For this review, take the finished solid that the model builds, in its own axes (mm). A direction names the side the tool comes from. Round coordinates to 2 decimals unless told otherwise and drop trailing zeros. Write each loop counter-clockwise with the first axis right and the second up, starting at its lowest first coordinate (ties: lowest second). Pieces come first, ordered by that corner, then holes. Notation, with made-up numbers: (65, 82.25) - (115, 82.25) arc R29 ccw to (115, 120.25) - close; hole circle Ø4 at (-8.75, 4). An arc over 180 degrees is marked (long way). One line per item, written item: value. Start each with the question number.
Q1. Add section B-B on x = -2.25. Write out the cut boundary in (y, z), and give its area (3 significant figures).
Q2. Tool access review of faces 4 (the face through (0, 0, -30)), 5 (the face through (0, 30, -60)): name each direction out of +Z, -Z, +X, -X, +Y, -Y from which nothing blocks a thin tool from reaching the whole face with its end or side.
Q3. For probe 1 along Y at (x, z) = (2, 0); probe 2 along Z at (x, y) = (-6, 80.5); probe 3 along Z at (x, y) = (-0.5, 57), list the stretches that pass through material, from the lowest coordinate up.
Q4. Mouldability with a two-part tool opening along Y and no side actions: class faces 1 (the face through (-6.35, 35, 28)), 2 (the face through (0.089, 119.985, -1.319)), 3 (the face through (-0.089, 80.275, 22.111)) as +Y half, -Y half, draft (parallel to the pull), parting line (faces both ways), or undercut.
Q5. Add section C-C on z = -10. Write out the cut boundary in (x, y).
Q6. Clearance check with flat-ended pins moving along their axes: pin 1 Ø1 at (x, y) = (-4, 81.5) entering from +Z (3 decimals); pin 2 Ø6.5 at (x, z) = (-0.5, -40) entering from -Y. State where each tip first meets the part, or that it passes through.
Q7. Add section D-D on z = 50. Write out the cut boundary in (x, y), and give its area (3 significant figures).
Q8. Add section A-A on y = 46.5. Write out the cut boundary in (x, z), and give its area (3 significant figures).
```python
from build123d import *

# Parameters (mm, degrees)
SKETCH1_R           = 30
BOSS_EXTRUDE1_DEPTH = 6.35


with BuildPart() as part:
    # Sketch1 → Boss-Extrude1 (new body, symmetric)
    with BuildSketch(Plane(origin=(0, 0, 0), x_dir=(0, 0, -1), z_dir=(1, 0, 0))):
        with BuildLine():
            Line((60, 0), (60, 60))
            ThreePointArc((60, 60), (0, 120), (-60, 60))
            Line((-60, 60), (-60, 0))
            Line((-60, 0), (-60, -20.621041836))
            ThreePointArc((-60, -20.621041836), (-31.722339788, -5.299116156), (0, 0))
            Line((0, 0), (60, 0))
        make_face()
        with Locations((0, 60)):
            Circle(SKETCH1_R, mode=Mode.SUBTRACT)
    extrude(amount=BOSS_EXTRUDE1_DEPTH, both=True)


solid = part.part
```
Result set:
1. outline: (-20.62, 60) arc R97.6 cw to (0, 0) - (0, -60) - (60, -60) arc R60 ccw to (60, 60) - close; hole circle Ø60 at (60, 0)
1. area: 10,400 mm^2
2. face 4: -Z, +X, -X, -Y
2. face 5: -Z, +X, -X, +Y, -Y
3. probe 1: y = 0 to 30, 90 to 120
3. probe 2: z = -56.39 to -21.9, 21.9 to 56.39
3. probe 3: z = -60 to -29.85, 29.85 to 60
4. face 1: draft
4. face 2: +Y half
4. face 3: undercut
5. outline: (-6.35, 0) - (6.35, 0) - (6.35, 31.72) - (-6.35, 31.72) - close; (-6.35, 88.28) - (6.35, 88.28) - (6.35, 119.16) - (-6.35, 119.16) - close
6. pin 1: stops at z = 56.205
6. pin 2: stops at y = 0
7. outline: (-6.35, -13.78) - (6.35, -13.78) - (6.35, 93.17) - (-6.35, 93.17) - close
7. area: 1,360 mm^2
8. outline: (-6.35, -60) - (6.35, -60) - (6.35, -26.79) - (-6.35, -26.79) - close; (-6.35, 26.79) - (6.35, 26.79) - (6.35, 60) - (-6.35, 60) - close
8. area: 844 mm^2
